from build123d import *

# Parameters (mm, degrees)
F0_R     = 6
F1_DEPTH = 52
F2_R     = 5.5
F3_DEPTH = 5
F4_R     = 4
F5_DEPTH = 2
F6_R     = 5
F7_DEPTH = 6.4


with BuildPart() as f1:
    # F0 (on Front) → F1 (new body)
    with BuildSketch(Plane.XZ):
        Circle(F0_R)
    extrude(amount=-F1_DEPTH)

    # F2 (on face) → F3 (join)
    with BuildSketch(Plane.XZ):
        Circle(F2_R)
    extrude(amount=F3_DEPTH)

    # F4 (on face) → F5 (join)
    with BuildSketch(Plane.XZ.offset(5)):
        Circle(F4_R)
    extrude(amount=F5_DEPTH)

    # F6 (on face) → F7 (join)
    with BuildSketch(Plane.XZ.offset(7)):
        Circle(F6_R)
    extrude(amount=F7_DEPTH)


solid = f1.part
Can you work these out from the model? Positions are in its coordinate system, mm. A direction names the side the tool comes from. Give positions to 0.01 mm unless a question says otherwise; leave off trailing zeros. Loops run counter-clockwise (first coordinate to the right, second up) from the corner with the lowest first, then second, coordinate; pieces in that order, holes last. Notation, with made-up numbers: M 6.25,-30.75 L 11.25,-30.75 A32 cw 11.25,0.25 Z; hole C 62.5,15.25 d8. An arc over 180 degrees is marked long. One line per item, written item: value.
1) On a 3-axis mill with a long thin cutter (end or side, diameter ignored), from which of +Z, -Z, +X, -X, +Y, -Y can I reach the whole of each face in a straight line? I mean faces 5 (the face through (-4, -5, -2)), 6 (the face through (0, -13.4, 0)), 7 (the face through (-1.19, -2.46, -5.37)). Say none if no direction works.
Geometry check:
face 5: none
face 6: +Z, -Z, +X, -X, -Y
face 7: -Y
2) Imagine slicing it at B-B on x = 0. Write out the boundary of the cut face in (y, z).
Geometry check:
outline: M -13.4,-5 L -7,-5 L -7,-4 L -5,-4 L -5,-5.5 L 0,-5.5 L 0,-6 L 52,-6 L 52,6 L 0,6 L 0,5.5 L -5,5.5 L -5,4 L -7,4 L -7,5 L -13.4,5 Z
3) Please list where these lines run through material, in increasing order: line 1 (Y direction, x = 2, z = 4.5); line 2 (Y direction, x = 4.25, z = -3.75); line 3 (Z direction, x = -1, y = 43).
Geometry check:
line 1: y = -13.4 to -7, -5 to 52
line 2: y = 0 to 52
line 3: z = -5.92 to 5.92
4) Thinking about a two-plate mould opening in Y: for faces 1 (the face through (-0.867, -5.986, -3.905)), 2 (the face through (-6, 26, 0)), 3 (the face through (3, 0, -5)), 4 (the face through (0, 52, 0)), which applies, +Y half, -Y half, draft (parallel to the pull), parting line (faces both ways), or undercut?
Geometry check:
face 1: undercut
face 2: draft
face 3: -Y half
face 4: +Y half
5) Imagine slicing it at A-A on z = 0. Write out the boundary of the cut face in (x, y), and give its area (3 significant figures).
Geometry check:
outline: M -6,0 L -5.5,0 L -5.5,-5 L -4,-5 L -4,-7 L -5,-7 L -5,-13.4 L 5,-13.4 L 5,-7 L 4,-7 L 4,-5 L 5.5,-5 L 5.5,0 L 6,0 L 6,52 L -6,52 Z
area: 759 mm²
